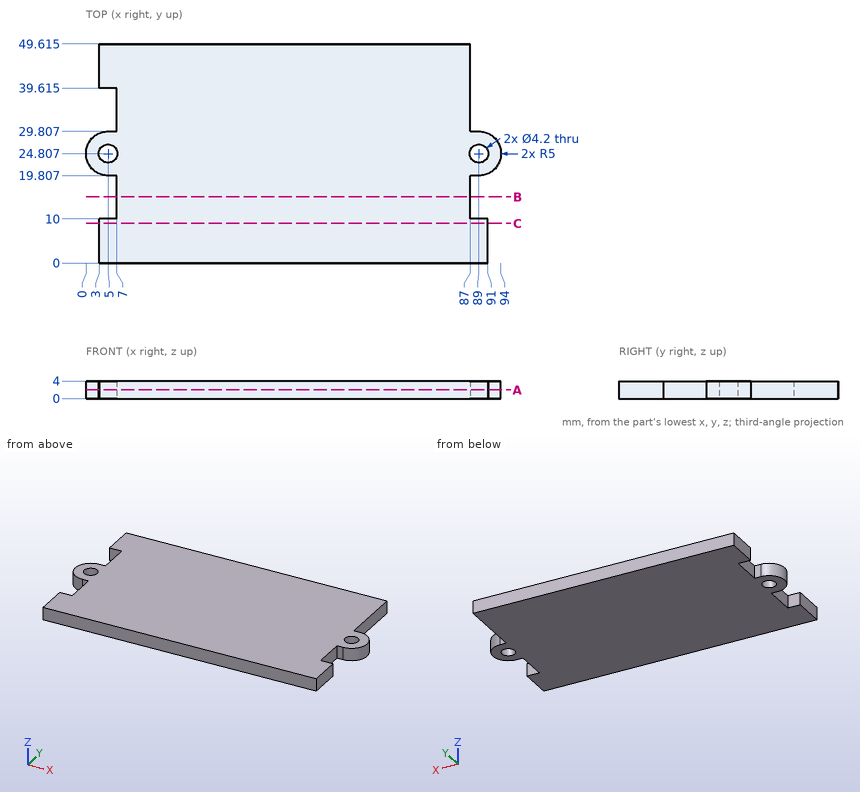
Geometry check sheet. Reference: drawing and pictorial views, mm from the part's lowest x, y, z. Round coordinates to 2 decimals unless told otherwise and drop trailing zeros. Order: outer loops, then holes, each group sorted by start corner. A loop starts at its lowest first (then second) coordinate and runs counter-clockwise, first axis right, second up. Notation, with made-up numbers: (-15, 88.5) - (12, 88.5) arc R6 cw to (12, 99.5) - close; hole circle Ø1 at (-37, -14). An arc over 180 degrees is marked (long way). One line per question, with ' | ' between items. Start each with the question number.
(1) Sectioned sample at C-C on y = 9. Record the cut outline in (x, z), and give its area (3 significant figures).
(2) Depth check by flat-ended pin: pin 1 Ø2 at (y, z) = (3.5, 1.5) entering from -X; pin 2 Ø1.2 at (x, z) = (88, 2.5) entering from +Y; pin 3 Ø1.2 at (y, z) = (16, 1) entering from -X. Enter the tip coordinate at first touch or a pass-through.
(3) Thickness scan on L1, parallel to Y at x = 89, z = 1.65; L2, parallel to X at y = 25, z = 0.8; L3, parallel to Y at x = 88.5, z = 1.75. Record the ranges inside material, lowest first. Write a range as [from, to].
(4) Sectioned sample at A-A on z = 2. Record the cut outline in (x, y) (1 decimal).
(5) Sectioned sample at B-B on y = 15. Record the cut outline in (x, z), and give its area (3 significant figures).
Conclusion:
1) outline: (3, 0) - (91, 0) - (91, 4) - (3, 4) - close | area: 352 mm2
2) pin 1: stops at x = 3 | pin 2: stops at y = 29.81 | pin 3: stops at x = 7
3) L1: y = [0, 10], [19.81, 22.71], [26.91, 29.81] | L2: x = [0, 2.91], [7.09, 86.91], [91.09, 94] | L3: y = [0, 10], [19.81, 22.77], [26.85, 29.81]
4) outline: (3, 0) - (91, 0) - (91, 10) - (87, 10) - (87, 19.8) - (89, 19.8) arc R5 ccw to (89, 29.8) - (87, 29.8) - (87, 49.6) - (3, 49.6) - (3, 39.6) - (7, 39.6) - (7, 29.8) - (5, 29.8) arc R5 ccw to (5, 19.8) - (7, 19.8) - (7, 10) - (3, 10) - close; hole circle Ø4.2 at (5, 24.8); hole circle Ø4.2 at (89, 24.8)
5) outline: (7, 0) - (87, 0) - (87, 4) - (7, 4) - close | area: 320 mm2
